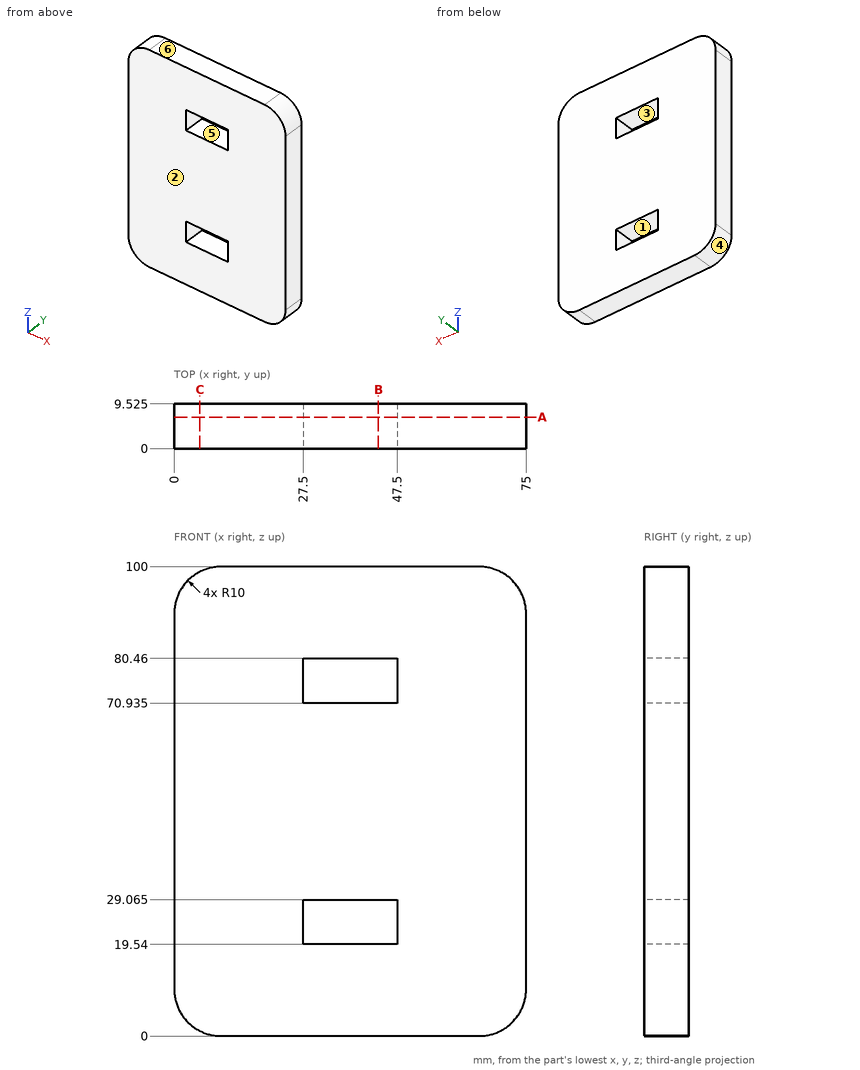
Geometry check sheet. Reference: drawing and pictorial views, mm from the part's lowest x, y, z. A direction names the side the tool comes from. Give positions to 0.01 mm unless a question says otherwise; leave off trailing zeros. Order: outer loops, then holes, each group sorted by start corner. A loop starts at its lowest first (then second) coordinate and runs counter-clockwise, first axis right, second up. Notation, with made-up numbers: M 83.5,-30.75 L 122.5,-30.75 A15 ccw 122.5,-18.75 Z; hole C 67.5,4 d8. An arc over 180 degrees is marked long. Return JSON: item names as keys, results as strings. Group by question number.
1) Section check B-B on x = 43.5. Record the cut outline in (y, z) (3 decimals), and give its area (3 significant figures).
2) Mould release check, pull along X, two halves, no side actions. Record for the marked faces 3, 4, 5 and 6: pulls with the +X half, pulls with the -X half, needs draft (parallel to the pull), parting line crosses it, or undercut.
3) Section check C-C on x = 5.5. Record the cut outline in (y, z) (3 decimals).
4) Section check A-A on y = 6.75. Record the cut outline in (x, z) (3 decimals), and give its area (3 significant figures).
5) Access from +Z, -Z, +X, -X, +Y, -Y to the whole of each face (thin tool, end or side, straight path). Record for the marked faces 1 and 2.
6) Scan lines: line 1 (X direction, y = 3, z = 72.5); line 2 (Z direction, x = 42, y = 3.75) (3 decimals); line 3 (X direction, y = 2, z = 8). Record each from-to range of solid material in increasing order.
Answer block:
{
 "1": {"outline": "M 0,0 L 9.525,0 L 9.525,19.54 L 0,19.54 Z; M 0,29.065 L 9.525,29.065 L 9.525,70.935 L 0,70.935 Z; M 0,80.46 L 9.525,80.46 L 9.525,100 L 0,100 Z", "area": "771 mm^2"},
 "2": {"face 3": "undercut", "face 4": "pulls with the -X half", "face 5": "undercut", "face 6": "needs draft"},
 "3": {"outline": "M 0,1.07 L 9.525,1.07 L 9.525,98.93 L 0,98.93 Z"},
 "4": {"outline": "M 0,10 A10 ccw 10,0 L 65,0 A10 ccw 75,10 L 75,90 A10 ccw 65,100 L 10,100 A10 ccw 0,90 Z; hole M 27.5,19.54 L 47.5,19.54 L 47.5,29.065 L 27.5,29.065 Z; hole M 27.5,70.935 L 47.5,70.935 L 47.5,80.46 L 27.5,80.46 Z", "area": "7,030 mm^2"},
 "5": {"face 1": "+Y, -Y", "face 2": "+Z, -Z, +X, -X, -Y"},
 "6": {"line 1": "x = 0 to 27.5, 47.5 to 75", "line 2": "z = 0 to 19.54, 29.065 to 70.935, 80.46 to 100", "line 3": "x = 0.2 to 74.8"}
}
